Autodesk Inventor part; units mm, degrees
ref_plane "YZ Plane" through (0, 0, 0) normal (1, 0, 0) x (0, 1, 0)
ref_plane "XZ Plane" through (0, 0, 0) normal (0, 1, 0) x (-1, 0, 0)
ref_plane "XY Plane" through (0, 0, 0) normal (0, 0, 1) x (1, 0, 0)
sketch "Sketch1" plane through (0, 0, 0) normal (0, 1, 0) x (-1, 0, 0)
  line L0 (-12.7, -12.7) -> (12.7, -12.7)
  line L1 (12.7, -12.7) -> (12.7, 12.7)
  line L2 (12.7, 12.7) -> (-12.7, 12.7)
  line L3 (-12.7, 12.7) -> (-12.7, -12.7)
  line L4 (-12.7, -12.7) -> (12.7, 12.7) construction
  line L5 (12.7, -12.7) -> (-12.7, 12.7) construction
  line L6 (-9.525, 9.525) -> (9.525, 9.525)
  line L7 (9.525, 9.525) -> (9.525, -9.525)
  line L8 (9.525, -9.525) -> (-9.525, -9.525)
  line L9 (-9.525, -9.525) -> (-9.525, 9.525)
  point P0 (0, 0)
  dimension "d0" = 25.4
  dimension "d1" = 25.4
  dimension "d2" = 3.175
extrude "Extrusion1" add sketch "Sketch1" along normal blind 279.4
sketch "Sketch2" plane through (-12.7, 0, -12.7) normal (-1, 0, 0) x (0, 0, 1)
  line L0 (22.225, 279.4) -> (3.175, 279.4)
  line L1 (12.7, 279.4) -> (12.7, 145.6182) construction
  line L2 (12.7, 0) -> (12.7, 29.845) construction
  circle A0 centre (12.7, 145.6182) radius 3.2512
  circle A1 centre (12.7, 29.845) radius 3.2512
  line L3 (12.7, 0) -> (12.7, 53.467) construction
  circle A2 centre (12.7, 53.467) radius 3.2512
  line L4 (0, 0) -> (25.4, 0) construction
  dimension "d5" = 6.5024
  dimension "d6" = 133.7818
  dimension "d7" = 6.5024
  dimension "d8" = 29.845
  dimension "d11" = 53.467
  dimension "d12" = 6.5024
extrude "Extrusion2" cut sketch "Sketch2" against normal blind 25.4 contours A0 | A1
extrude "Extrusion3" cut sketch "Sketch2" against normal blind 25.4 contours A2
properties part number "STRU_023_Kenji_11in" material "Aluminum 6061"
Geometry check sheet. Reference: the model listing, model coordinates, mm. A direction names the side the tool comes from. Round coordinates to 2 decimals unless told otherwise and drop trailing zeros. Loops run counter-clockwise (first coordinate to the right, second up) from the corner with the lowest first, then second, coordinate; pieces in that order, holes last. Notation, with made-up numbers: (67, 89) -> (90, 89) arc R9 cw to (90, 100) -> close; hole circle Ø5 at (64.25, 0.5). An arc over 180 degrees is marked (long way). Use a Markdown table: item, result.
(1) Set-up check for faces 5 (the cylindrical face through (11.09, 142.444, -0.705)), 6 (the flat face through (9.525, 138, 0)): record each of +Z, -Z, +X, -X, +Y, -Y from which the full face is reachable in a straight line by a thin tool's end or side.
Calculated:
| item | result |
|---|---|
| face 5 | +X, -X |
| face 6 | +Y, -Y |
(2) Scan lines: probe 1 along Y at (x, z) = (-10.85, 0); probe 2 along X at (y, z) = (216.5, 0.25) (3 decimals). Record each from-to range of solid material in increasing order.
Calculated:
| item | result |
|---|---|
| probe 1 | 0 to 26.59, 33.1 to 50.22, 56.72 to 142.37, 148.87 to 279.4 |
| probe 2 | -12.7 to -9.525, 9.525 to 12.7 |
(3) Sectioned sample at C-C (y = 94). Enter the section's corners in (x, z) (3 decimals).
Calculated:
| item | result |
|---|---|
| outline | (-12.7, -12.7) -> (12.7, -12.7) -> (12.7, 12.7) -> (-12.7, 12.7) -> close; hole (-9.525, -9.525) -> (9.525, -9.525) -> (9.525, 9.525) -> (-9.525, 9.525) -> close |
(4) Mould release check, pull along X, two halves, no side actions. Record for faces 1 (the flat face through (0, 138, -9.525)), 2 (the flat face through (-9.525, 138, 0)), 3 (the flat face through (12.7, 138, 0)), 4 (the cylindrical face through (-11.13, 56.69, -0.42)): released by +X, released by -X, zero draft, split by the parting line, or undercut.
Calculated:
| item | result |
|---|---|
| face 1 | undercut |
| face 2 | undercut |
| face 3 | released by +X |
| face 4 | zero draft |
(5) Sectioned sample at A-A (z = 0). Give the number of separate pieces and of enclosed holes in the cut face, then the cut area to 3 significant figures.
Calculated:
| item | result |
|---|---|
| separate pieces | 8 |
| enclosed holes | 0 |
| area | 1,650 mm² |
(6) Go/stop test with a flat-tipped pin: P1, Ø4, axis at y = 53.467, z = 0, coming from the +X side. Record where the tip stops, or that it passes through.
Calculated:
| item | result |
|---|---|
| P1 | through |
(7) Sectioned sample at B-B (x = -1.75). Enter the section's corners in (y, z) (3 decimals).
Calculated:
| item | result |
|---|---|
| outline | (0, -12.7) -> (279.4, -12.7) -> (279.4, -9.525) -> (0, -9.525) -> close; (0, 9.525) -> (279.4, 9.525) -> (279.4, 12.7) -> (0, 12.7) -> close |
